Source: CAD feature listing. Evaluate the final solid. Frame: model axes, mm. Face numbers are marked on the shaded views. Give positions to 0.01 mm unless a question says otherwise; leave off trailing zeros. Write each loop counter-clockwise with the first axis right and the second up, starting at its lowest first coordinate (ties: lowest second). Pieces come first, ordered by that corner, then holes. Notation, with made-up numbers: M -9.75,13 L 27.25,13 A15 ccw 27.25,42 Z; hole C 82,65 d11. An arc over 180 degrees is marked long. Answer as a JSON object with one key per item and string values. Group by question number.
Autodesk Fusion 360 part; units mm, degrees
sketch "Sketch1" plane through (0, 0, 0) normal (0, 0, 1) x (1, 0, 0)
  line L0 (21, 6) -> (-21, 6)
  line L1 (-21, 6) -> (-21, -6)
  line L2 (-21, -6) -> (21, -6)
  line L3 (21, -6) -> (21, 6)
  line L4 (21, 6) -> (-21, -6) construction
  line L5 (-21, 6) -> (21, -6) construction
  line L6 (-16, 0) -> (16, 0) construction
  circle A0 centre (-16, 0) radius 2.35
  circle A1 centre (16, 0) radius 2.35
  dimension "d1" = 12
  dimension "d2" = 42
  dimension "d3" = 32
  dimension "d4" = 4.7
extrude "Extrude1" add sketch "Sketch1" along normal blind 3 contours L0 L1 L2 L3 | A0 | A1
sketch "Sketch2" plane through (0, 0, 3) normal (0, 0, 1) x (-1, 0, 0)
  line L0 (-21, 6) -> (-21, -6)
  line L1 (-21, -6) -> (21, -6)
  line L2 (21, -6) -> (21, 6)
  line L3 (21, 6) -> (-21, 6)
  line L4 (16, 0) -> (-16, 0) construction
  circle A0 centre (16, 0) radius 1.5
  circle A1 centre (-16, 0) radius 1.5
  dimension "d7" = 32
  dimension "d11" = 3
extrude "Extrude2" add sketch "Sketch2" along normal blind 2 contours A0 | A1
sketch "Sketch3" plane through (0, 0, 3) normal (0, 0, 1) x (-1, 0, 0)
  line L0 (12, 2.5) -> (-12, 2.5)
  line L1 (-12, 2.5) -> (-12, -2.5)
  line L2 (-12, -2.5) -> (12, -2.5)
  line L3 (12, -2.5) -> (12, 2.5)
  line L4 (12, 2.5) -> (-12, -2.5) construction
  line L5 (-12, 2.5) -> (12, -2.5) construction
  dimension "d14" = 24
  dimension "d15" = 5
extrude "Extrude3" cut sketch "Sketch3" against normal blind 2
sketch "Sketch4" plane through (0, 0, 0) normal (0, 1, 0) x (1, 0, 0)
  line L0 (14.5, -5) -> (17.5, -5)
  line L1 (17.5, -3) -> (14.5, -3)
  line L2 (17.5, -3) -> (17.5, -5)
  line L3 (14.5, -3) -> (14.5, -5)
  line L4 (17.5, -4.2) -> (17.9619, -5)
  line L5 (17.9619, -5) -> (16, -7.8019)
  line L6 (16, -5) -> (16, -7.8019)
  line L7 (0, 0) -> (0, -0.3324)
  line L8 (0, -0.3324) -> (0, -9.743) construction
  line L9 (-17.9619, -5) -> (-16, -7.8019)
  line L10 (-17.5, -4.2) -> (-17.9619, -5)
  line L11 (-16, -5) -> (-16, -7.8019)
  line L12 (-17.5, -5) -> (-14.5, -5)
  line L13 (-14.5, -3) -> (-17.5, -3)
  line L14 (-17.5, -3) -> (-17.5, -5)
  line L15 (16, -7.8019) -> (14.0381, -5)
  arc A0 (14.3617, -5.4621) -> (17.6383, -5.4621) centre (16, -4.315) ccw
  arc A1 (-17.6383, -5.4621) -> (-14.3617, -5.4621) centre (-16, -4.315) ccw
  point P0 (16, -6.315)
  dimension "d19" = 1.2
  dimension "d22" = 30
  dimension "d23" = 2
  dimension "d27" = 2
  dimension "d29" = 70
revolve "Revolve1" add sketch "Sketch4" angle 360 about axis through (16, 0, 5) along (0, 0, 1) contours L0 L2 L4 L5 L6 A0
revolve "Revolve2" add sketch "Sketch4" angle 360 about axis through (-16, 0, 5) along (0, 0, 1) contours L9 L10 L11 L12 L14 A1
fillet "Fillet1" radius 0.4 2 edges at (14.1709, -0.7094, 5) (-17.8291, 0.7094, 5)
sketch "Sketch5" plane through (0, 0, 3) normal (0, 0, 1) x (-1, 0, 0)
  line L0 (-12, 2.5) -> (12, 2.5)
  line L1 (12, 2.5) -> (12, -2.5)
  line L2 (12, -2.5) -> (-12, -2.5)
  line L3 (-12, -2.5) -> (-12, 2.5)
  circle A0 centre (-16, 0) radius 1.5 construction
  circle A1 centre (16, 0) radius 1.5 construction
  line L4 (-21, 6) -> (-21, -6)
  line L5 (-21, -6) -> (21, -6)
  line L6 (21, -6) -> (21, 6)
  line L7 (21, 6) -> (-21, 6)
  circle A2 centre (16, 0) radius 1.8157 construction
  circle A3 centre (-16, 0) radius 1.8157 construction
  line L8 (15.6, 3.5) -> (16.4, 3.5)
  line L9 (16.4, 3.5) -> (16.4, -3.5)
  line L10 (16.4, -3.5) -> (15.6, -3.5)
  line L11 (15.6, -3.5) -> (15.6, 3.5)
  line L12 (15.6, 3.5) -> (16.4, -3.5) construction
  line L13 (16.4, 3.5) -> (15.6, -3.5) construction
  line L14 (-16.4, 3.5) -> (-15.6, 3.5)
  line L15 (-15.6, 3.5) -> (-15.6, -3.5)
  line L16 (-15.6, -3.5) -> (-16.4, -3.5)
  line L17 (-16.4, -3.5) -> (-16.4, 3.5)
  line L18 (-16.4, 3.5) -> (-15.6, -3.5) construction
  line L19 (-15.6, 3.5) -> (-16.4, -3.5) construction
  point P0 (16, 0)
  point P1 (-16, 0)
  dimension "d32" = 7
  dimension "d33" = 0.8
extrude "Extrude4" cut sketch "Sketch5" along normal blind 10 contours L8 L9 L10 L11 | L14 L15 L16 L17
fillet "Fillet2" radius 1 4 edges at (21, -6, 1.5) (-21, -6, 1.5) (-21, 6, 1.5) (21, 6, 1.5)
chamfer "Chamfer1" distance 0.6 angle 45 8 edges at (0, -6, 0) (20.7071, -5.7071, 0) (21, 0, 0) (20.7071, 5.7071, 0) (0, 6, 0) (-20.7071, 5.7071, 0) (-21, 0, 0) (-20.7071, -5.7071, 0)
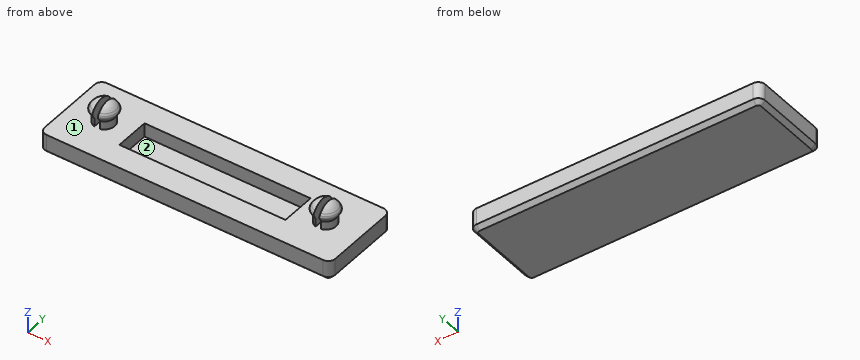
(1) Contact query for flat-ended pins moving along their axis: pin 1 Ø3.5 at (y, z) = (0, 5.5) entering from -X; pin 2 Ø2.5 at (x, y) = (1.5, -1) entering from +Z; pin 3 Ø3.5 at (y, z) = (0, 4) entering from +X; pin 4 Ø1 at (y, z) = (0.5, 5) entering from +X. Output: stop coordinate, or through.
(2) Section C-C, the plane x = 2. Return loops of the section in (y, z).
(3) Section D-D, the plane y = 3.25. Return loops of the section in (x, z), plus the area to 3 significant figures.
(4) Ray query, L1, parallel to X at y = 0.75, z = 4.5; L2, parallel to X at y = -1.75, z = 2; L3, parallel to X at y = 1.25, z = 4.25. Return the intervals inside material, ascending. Write a range as [from, to].
(5) Section A-A, the plane z = 3.5. Return loops of the section in (x, y).
(6) Pull-direction query (Y, two-part tool) for the marked faces 1 and 2; classes: pulls with the +Y half, pulls with the -Y half, needs draft (parallel to the pull), parting line crosses it, or undercut.
(7) Section B-B, the plane z = 1.5. Return loops of the section in (x, y).
Reported:
{
 "1": {"pin 1": "stops at x = -17.89", "pin 2": "stops at z = 1", "pin 3": "stops at x = 21", "pin 4": "stops at x = 17.89"},
 "2": {"outline": "M -6,0.6 L -5.4,0 L 5.4,0 L 6,0.6 L 6,3 L 2.5,3 L 2.5,1 L -2.5,1 L -2.5,3 L -6,3 Z"},
 "3": {"outline": "M -21,0.6 L -20.4,0 L 20.4,0 L 21,0.6 L 21,3 L -21,3 Z", "area": "126 mm2"},
 "4": {"L1": "x = [-17.5, -16.4], [-15.6, -14.5], [14.5, 15.6], [16.4, 17.5]", "L2": "x = [-21, -12], [12, 21]", "L3": "x = [-16.88, -16.4], [-15.6, -15.12], [15.12, 15.6], [16.4, 16.88]"},
 "5": {"outline": "M -16.4,-1.45 L -16.4,1.45 A1.5 ccw Z; M -15.6,-1.45 A1.5 ccw -15.6,1.45 Z; M 15.6,-1.45 L 15.6,1.45 A1.5 ccw Z; M 16.4,-1.45 A1.5 ccw 16.4,1.45 Z"},
 "6": {"face 1": "needs draft", "face 2": "undercut"},
 "7": {"outline": "M -21,-5 A1 ccw -20,-6 L 20,-6 A1 ccw 21,-5 L 21,5 A1 ccw 20,6 L -20,6 A1 ccw -21,5 Z; hole M -12,-2.5 L 12,-2.5 L 12,2.5 L -12,2.5 Z"}
}
